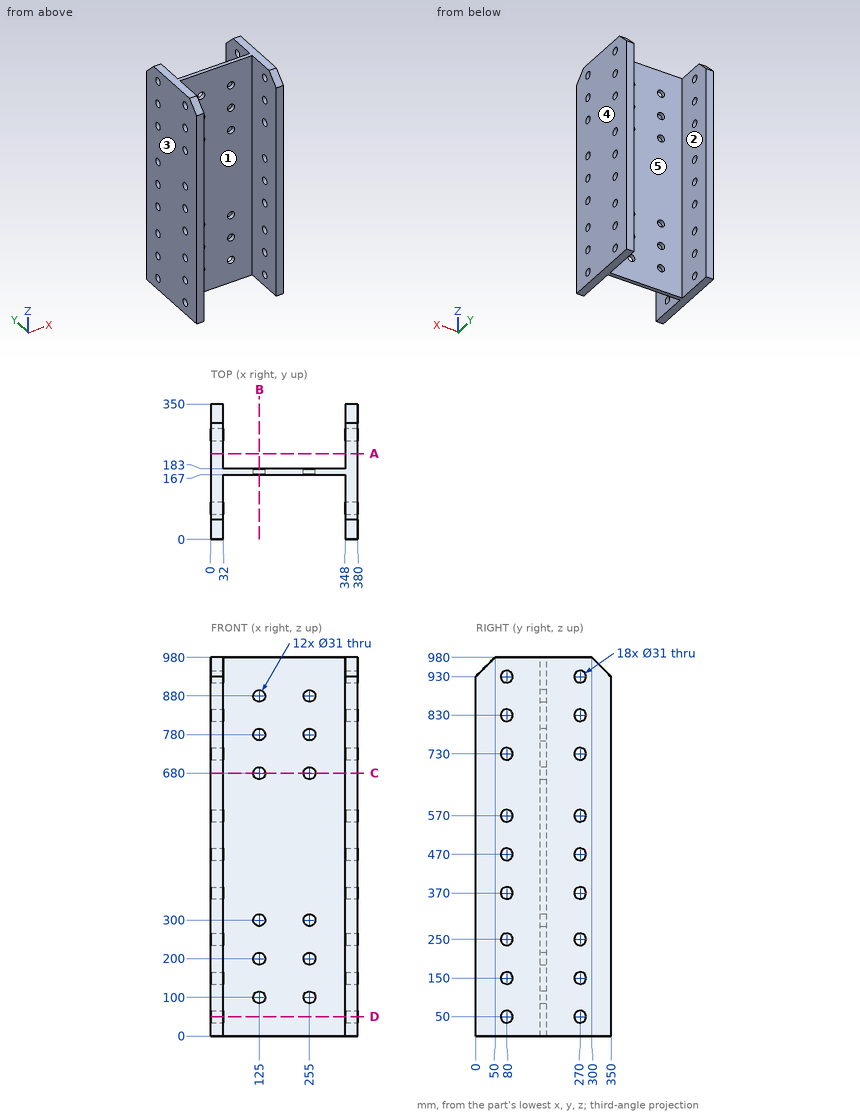
The figure shows three views and two pictorial views of one solid part (mm, origin at its lowest corner). Answer the questions. A direction names the side the tool comes from. Coordinates: 2 decimals unless noted, no trailing zeros. Loops run counter-clockwise (first coordinate to the right, second up) from the corner with the lowest first, then second, coordinate; pieces in that order, holes last. Notation, with made-up numbers: (-37.5, -37) - (-30.5, -37) arc R14 cw to (-30.5, -29) - close; hole circle Ø6 at (11.5, 47). An arc over 180 degrees is marked (long way). Write item = value, one per line.
1) Section D-D (z = 50) is taken. Determine the outline of the cut face in (x, y).
Responses:
outline = (0, 0) - (32, 0) - (32, 64.5) - (0, 64.5) - close; (0, 95.5) - (32, 95.5) - (32, 167) - (348, 167) - (348, 95.5) - (380, 95.5) - (380, 254.5) - (348, 254.5) - (348, 183) - (32, 183) - (32, 254.5) - (0, 254.5) - close; (0, 285.5) - (32, 285.5) - (32, 350) - (0, 350) - close; (348, 0) - (380, 0) - (380, 64.5) - (348, 64.5) - close; (348, 285.5) - (380, 285.5) - (380, 350) - (348, 350) - close
2) Which of the six approach directions +Z, -Z, +X, -X, +Y, -Y give full straight-line access (tool end or side, diameter ignored) to the marked faces 1 and 2?
Responses:
face_1 = +Z, -Z, -Y
face_2 = +Z, -Z, +Y
3) Section C-C (z = 680) is taken. Determine the outline of the cut face in (x, y).
Responses:
outline = (0, 0) - (32, 0) - (32, 167) - (109.5, 167) - (109.5, 183) - (32, 183) - (32, 350) - (0, 350) - close; (140.5, 167) - (239.5, 167) - (239.5, 183) - (140.5, 183) - close; (270.5, 167) - (348, 167) - (348, 0) - (380, 0) - (380, 350) - (348, 350) - (348, 183) - (270.5, 183) - close
4) This flat-tipped pin is pushed along its axis until it touches: P1, Ø6, axis at x = 252.5, z = 617.5, coming from the -Y side. Where does it stop, or does it pass through?
Responses:
P1 = 167
5) Find the intervals of material crossed by line 1 along X through (y, z) = (172.5, 680); line 2 along X through (y, z) = (302.5, 475); line 3 along Y through (x, z) = (16, 726), in increasing order.
Responses:
line_1 = 0 to 109.5, 140.5 to 239.5, 270.5 to 380
line_2 = 0 to 32, 348 to 380
line_3 = 0 to 65.03, 94.97 to 255.03, 284.97 to 350
6) Section B-B (x = 125) is taken. Determine the outline of the cut face in (y, z).
Responses:
outline = (167, 0) - (183, 0) - (183, 84.5) - (167, 84.5) - close; (167, 115.5) - (183, 115.5) - (183, 184.5) - (167, 184.5) - close; (167, 215.5) - (183, 215.5) - (183, 284.5) - (167, 284.5) - close; (167, 315.5) - (183, 315.5) - (183, 664.5) - (167, 664.5) - close; (167, 695.5) - (183, 695.5) - (183, 764.5) - (167, 764.5) - close; (167, 795.5) - (183, 795.5) - (183, 864.5) - (167, 864.5) - close; (167, 895.5) - (183, 895.5) - (183, 980) - (167, 980) - close
7) Section A-A (y = 221.5) is taken. Determine the outline of the cut face in (x, z), plus the area to 3 significant figures.
Responses:
outline = (0, 0) - (32, 0) - (32, 980) - (0, 980) - close; (348, 0) - (380, 0) - (380, 980) - (348, 980) - close
area = 62,700 mm^2
8) Determine the mould class of the marked faces 3, 4 and 5 for opening direction X: pulls with the +X half, pulls with the -X half, needs draft (parallel to the pull), parting line crosses it, or undercut.
Responses:
face_3 = pulls with the -X half
face_4 = pulls with the +X half
face_5 = undercut
